Autodesk Inventor part; units mm, degrees
ref_plane "YZ Plane" through (0, 0, 0) normal (1, 0, 0) x (0, 1, 0)
ref_plane "XZ Plane" through (0, 0, 0) normal (0, 1, 0) x (-1, 0, 0)
ref_plane "XY Plane" through (0, 0, 0) normal (0, 0, 1) x (1, 0, 0)
sketch "Эскиз1" plane through (0, 0, 0) normal (0, 0, 1) x (1, 0, 0)
  circle A0 centre (25, -25) radius 1.75
  circle A1 centre (25, 25) radius 1.75
  line L0 (20.6111, 32.2931) -> (30.5924, 32.2931)
  line L1 (30.4739, -29.2685) -> (20.6111, -29.2685)
  line L2 (40.1458, 7.8878) -> (58.5047, 7.8878)
  line L3 (58.5047, 7.8878) -> (58.5047, -21.7573)
  line L4 (58.5047, -21.7573) -> (34.0362, -21.7573)
  arc A2 (29.5, 0) -> (20.6111, 21.1053) centre (0, 0) ccw
  arc A3 (20.6111, -21.1053) -> (29.5, 0) centre (0, 0) ccw
  line L5 (30.5924, 32.2931) -> (40.1458, 7.8878)
  line L6 (30.4739, -29.2685) -> (34.0362, -21.7573)
  line L7 (20.6111, -29.2685) -> (20.6111, -21.1053)
  line L8 (20.6111, 21.1053) -> (20.6111, 32.2931)
  line L9 (25, 25) -> (25, -25) construction
  line L10 (25, 0) -> (58.5047, 0) construction
  dimension "d10" = 25
  dimension "d11" = 25
extrude "Выдавливание1" add sketch "Эскиз1" along normal blind 1.5
fillet "Сопряжение1" radius 5 10 edges at (20.6111, -29.2685, 0.75) (20.6111, 32.2931, 0.75) (20.6111, -21.1053, 0.75) (20.6111, 21.1053, 0.75) (30.5924, 32.2931, 0.75) (40.1458, 7.8878, 0.75) (34.0362, -21.7573, 0.75) (58.5047, -21.7573, 0.75) (58.5047, 7.8878, 0.75) (30.4739, -29.2685, 0.75)
sketch "Эскиз2" plane through (0, 0, 1.5) normal (0, 0, 1) x (1, 0, 0)
  line L0 (55.5047, 2.0132) -> (55.5047, -17.9868)
  line L1 (55.5047, -17.9868) -> (55.5047, 2.0132)
  circle A0 centre (55.5047, 2.0132) radius 1.5
  circle A1 centre (55.5047, -17.9868) radius 1.5
  line L2 (58.5047, 2.8878) -> (58.5047, -16.7573)
  line L3 (58.5047, -16.7573) -> (58.5047, 2.8878)
  line L4 (58.5047, -7.9868) -> (55.5047, -7.9868)
  point P0 (0, 0)
  dimension "d4" = 3
  dimension "d5" = 3
  dimension "d6" = 3
  dimension "d7" = 20
extrude "Выдавливание2" cut sketch "Эскиз2" against normal blind 1.5
properties part number "крепление вентилятора1"
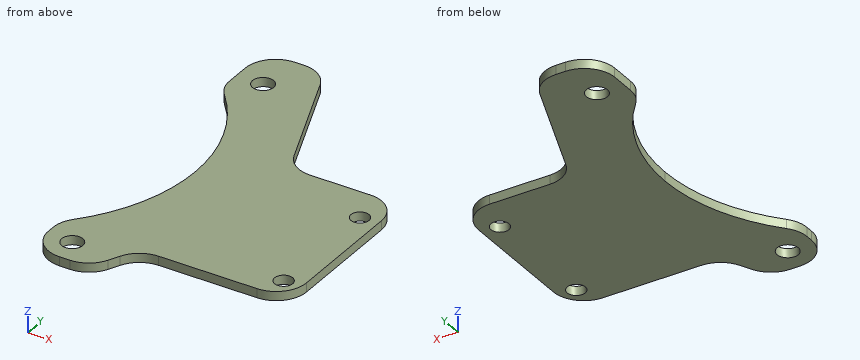
The listing builds one solid part. Answer for the finished solid, in the listing's coordinates (mm). Coordinates: 2 decimals unless noted, no trailing zeros. Loops run counter-clockwise (first coordinate to the right, second up) from the corner with the lowest first, then second, coordinate; pieces in that order, holes last. Notation, with made-up numbers: (-17, 62) -> (-13, 62) arc R23 ccw to (-13, 79) -> close; hole circle Ø7 at (-40, -11.5). An arc over 180 degrees is marked (long way). Answer in a Markdown table with one row per item. Add a question column.
1. A flat-ended cylindrical pin translates along its axis: P1, Ø3.5, axis at x = 55.5, y = 2.01, coming from the -Z side. Find the tip coordinate at first contact, or state that the pin passes through.
2. The part is cut by section A-A, the plane x = 25. Write down the section's boundary in (y, z).
3. The part is cut by section B-B, the plane y = 25. Write down the section's boundary in (x, z), then the cut area to 3 significant figures.
4. The part is cut by section C-C, the plane z = 0.35. Write down the section's boundary in (x, y), then the cut area to 3 significant figures.
5. The part is cut by section D-D, the plane x = 55.5. Write down the section's boundary in (y, z), then the cut area to 3 significant figures.
6. Consider line 1 (Y direction, x = 25, z = 0.95); line 2 (Y direction, x = 52, z = 0.7); line 3 (Y direction, x = 23, z = 0.7). Determine where each line is inside the solid, lowest interval first. Write a range as [from, to].
Answer below:
| question | item | result |
|---|---|---|
| 1 | P1 | z = 0 |
| 2 | outline | (-29.23, 0) -> (-26.75, 0) -> (-26.75, 1.5) -> (-29.23, 1.5) -> close; (-23.25, 0) -> (-15.66, 0) -> (-15.66, 1.5) -> (-23.25, 1.5) -> close; (15.66, 0) -> (23.25, 0) -> (23.25, 1.5) -> (15.66, 1.5) -> close; (26.75, 0) -> (32.26, 0) -> (32.26, 1.5) -> (26.75, 1.5) -> close |
| 3 | outline | (20.61, 0) -> (23.25, 0) -> (23.25, 1.5) -> (20.61, 1.5) -> close; (26.75, 0) -> (33.45, 0) -> (33.45, 1.5) -> (26.75, 1.5) -> close |
| 3 | area | 14.0 mm2 |
| 4 | outline | (20.61, -24.27) arc R5 ccw to (25.61, -29.27) -> (27.31, -29.27) arc R5 ccw to (31.83, -26.41) -> (32.68, -24.61) arc R5 cw to (37.2, -21.76) -> (53.5, -21.76) arc R5 ccw to (58.5, -16.76) -> (58.5, 2.89) arc R5 ccw to (53.5, 7.89) -> (43.56, 7.89) arc R5 cw to (38.9, 11.07) -> (31.84, 29.12) arc R5 ccw to (27.18, 32.29) -> (25.61, 32.29) arc R5 ccw to (20.61, 27.29) -> (20.61, 23.12) arc R5 ccw to (21.9, 19.77) arc R29.5 cw to (29.5, 0) arc R29.5 cw to (21.9, -19.77) arc R5 ccw to (20.61, -23.12) -> close; hole circle Ø3.5 at (25, -25); hole circle Ø3.5 at (25, 25); hole circle Ø3 at (55.5, -17.99); hole circle Ø3 at (55.5, 2.01) |
| 4 | area | 1,260 mm2 |
| 5 | outline | (-21.34, 0) -> (-19.49, 0) -> (-19.49, 1.5) -> (-21.34, 1.5) -> close; (-16.49, 0) -> (0.51, 0) -> (0.51, 1.5) -> (-16.49, 1.5) -> close; (3.51, 0) -> (7.47, 0) -> (7.47, 1.5) -> (3.51, 1.5) -> close |
| 5 | area | 34.2 mm2 |
| 6 | line 1 | [-29.23, -26.75], [-23.25, -15.66], [15.66, 23.25], [26.75, 32.26] |
| 6 | line 2 | [-21.76, 7.89] |
| 6 | line 3 | [-28.53, -18.47], [18.47, 31.56] |
